Here's how the part is built. I have some questions about the finished solid (model axes, mm). A direction names the side the tool comes from. Give positions to 0.01 mm unless a question says otherwise; leave off trailing zeros. Loops run counter-clockwise (first coordinate to the right, second up) from the corner with the lowest first, then second, coordinate; pieces in that order, holes last. Notation, with made-up numbers: (-21.75, 10.25) -> (8.25, 10.25) arc R15 cw to (8.25, 37.25) -> close; hole circle Ø10 at (11, -9). An arc over 180 degrees is marked (long way). Answer in a Markdown table with one row per item. Add a question column.
Item 1: If I drill on line 1 (X direction, y = -33, z = 5.25); line 2 (X direction, y = -3.5, z = 1); line 3 (Y direction, x = -84, z = 6.55), over which ranges is the centre line in solid material (lowest first)?
Item 2: If we section it at B-B (y = -34): Write out the boundary of the cut face in (x, z), then the cut area to 3 significant figures.
Item 3: For P1, Ø3, axis at x = -84, y = -34, coming from the -Z side; P2, Ø4.5, axis at x = -84, y = 34, coming from the +Z side, each with a flat end and sliding along its axis, tell me the tip position at first contact or that it passes through.
Item 4: If we section it at D-D (x = 40): Write out the boundary of the cut face in (y, z).
Item 5: If we section it at A-A (x = 0): Write out the boundary of the cut face in (y, z).
Item 6: Which directions (+Z, -Z, +X, -X, +Y, -Y) give clear straight access to the entire face, cutting with the end or side of a thin tool? Please do faces 1 (the face through (-81.33, -33.16, 6.03)), 2 (the face through (-37, 21.6, 2)), 3 (the face through (53, 0, 4)).
Item 7: If we section it at C-C (z = 6): Give the number of separate pieces and of enclosed holes in the cut face, then the cut area to 3 significant figures.
Item 8: We'd pull the mould along Y, two halves only. Please class faces 4 (the face through (-1, 1, 8)), 5 (the face through (-84, -36, 4)), 6 (the face through (-1, 38, 4)): released by +Y, released by -Y, zero draft, split by the parting line, or undercut.
```python
from build123d import *

# Parameters (mm, degrees)
SKETCH_1_W          = 176
SKETCH_1_H          = 76
EXTRUDE_1_DEPTH     = 8
SKETCH_2_R          = 1.6
CUT_EXTRUDE_1_DEPTH = 9
SKETCH_2_3_R        = 2.6
CUT_EXTRUDE_2_DEPTH = 3
SKETCH_4_R          = 2.8
CUT_EXTRUDE_3_DEPTH = 4
FILLET_1_R          = 2
SKETCH1_R           = 1.6
CUT_EXTRUDE1_DEPTH  = 9
SKETCH2_R           = 3
CUT_EXTRUDE2_DEPTH  = 4
CUT_EXTRUDE3_DEPTH  = 9


with BuildPart() as part:
    # 草图1 → 凸台-拉伸1 (new body)
    with BuildSketch(Plane.XY):
        Rectangle(SKETCH_1_W, SKETCH_1_H)
    extrude(amount=EXTRUDE_1_DEPTH)

    # 草图2 → 切除-拉伸1 (cut, through all)
    with BuildSketch(Plane(origin=(0, 0, 0), x_dir=(-1, 0, 0), z_dir=(0, 0, -1))):
        with Locations((-84, 34)):
            Circle(SKETCH_2_R)
        with Locations((0, 34)):
            Circle(SKETCH_2_R)
        with Locations((84, 34)):
            Circle(SKETCH_2_R)
        with Locations((-84, -34)):
            Circle(SKETCH_2_R)
        with Locations((84, -34)):
            Circle(SKETCH_2_R)
    extrude(amount=-CUT_EXTRUDE_1_DEPTH, mode=Mode.SUBTRACT)

    # 草图2<3> → 切除-拉伸2 (cut)
    with BuildSketch(Plane(origin=(0, 0, 0), x_dir=(-1, 0, 0), z_dir=(0, 0, -1))):
        with Locations((-84, 0)):
            Circle(SKETCH_2_3_R)
        with Locations((84, 0)):
            Circle(SKETCH_2_3_R)
        with Locations((0, -34)):
            Circle(SKETCH_2_3_R)
    extrude(amount=-CUT_EXTRUDE_2_DEPTH, mode=Mode.SUBTRACT)

    # 草图4 → 切除-拉伸3 (cut)
    with BuildSketch(Plane.XY.offset(8)):
        with Locations((-84, 34)):
            Circle(SKETCH_4_R)
        with Locations((0, 34)):
            Circle(SKETCH_4_R)
        with Locations((-84, -34)):
            Circle(SKETCH_4_R)
        with Locations((84, 34)):
            Circle(SKETCH_4_R)
        with Locations((84, -34)):
            Circle(SKETCH_4_R)
    extrude(amount=-CUT_EXTRUDE_3_DEPTH, mode=Mode.SUBTRACT)

    # 圆角1
    fillet_1_edges = [part.edges().sort_by_distance(p)[0] for p in [
        (-88, 38, 4),
        (88, 38, 4),
        (88, -38, 4),
        (-88, -38, 4),
    ]]
    fillet(fillet_1_edges, radius=FILLET_1_R)

    # Sketch1 → Cut-Extrude1 (cut, through all)
    with BuildSketch(Plane.XY.offset(8)):
        with Locations((-40, 21.5)):
            Circle(SKETCH1_R)
        with Locations((40, 21.5)):
            Circle(SKETCH1_R)
        with Locations((40, -21.5)):
            Circle(SKETCH1_R)
        with Locations((-40, -21.5)):
            Circle(SKETCH1_R)
    extrude(amount=-CUT_EXTRUDE1_DEPTH, mode=Mode.SUBTRACT)

    # Sketch2 → Cut-Extrude2 (cut)
    with BuildSketch(Plane(origin=(0, 0, 0), x_dir=(-1, 0, 0), z_dir=(0, 0, -1))):
        with Locations((-40, 21.5)):
            Circle(SKETCH2_R)
        with Locations((40, 21.5)):
            Circle(SKETCH2_R)
        with Locations((40, -21.5)):
            Circle(SKETCH2_R)
        with Locations((-40, -21.5)):
            Circle(SKETCH2_R)
    extrude(amount=-CUT_EXTRUDE2_DEPTH, mode=Mode.SUBTRACT)

    # Sketch3 → Cut-Extrude3 (cut, through all)
    with BuildSketch(Plane.XY.offset(8)):
        with BuildLine():
            Line((-73, -15), (-73, 15))
            ThreePointArc((-73, 15), (-63, 25), (-53, 15))
            Line((-53, 15), (-53, -15))
            ThreePointArc((-53, -15), (-63, -25), (-73, -15))
        make_face()
        with BuildLine():
            Line((73, -15), (73, 15))
            ThreePointArc((73, 15), (63, 25), (53, 15))
            Line((53, 15), (53, -15))
            ThreePointArc((53, -15), (63, -25), (73, -15))
        make_face()
    extrude(amount=-CUT_EXTRUDE3_DEPTH, mode=Mode.SUBTRACT)


solid = part.part
```
Recorded:
| question | item | result |
|---|---|---|
| 1 | line 1 | x = -88 to -86.62, -81.38 to 81.38, 86.62 to 88 |
| 1 | line 2 | x = -88 to -73, -53 to 53, 73 to 88 |
| 1 | line 3 | y = -38 to -36.8, -31.2 to 31.2, 36.8 to 38 |
| 2 | outline | (-88, 0) -> (-85.6, 0) -> (-85.6, 4) -> (-86.8, 4) -> (-86.8, 8) -> (-88, 8) -> close; (-82.4, 0) -> (-2.6, 0) -> (-2.6, 3) -> (2.6, 3) -> (2.6, 0) -> (82.4, 0) -> (82.4, 4) -> (81.2, 4) -> (81.2, 8) -> (-81.2, 8) -> (-81.2, 4) -> (-82.4, 4) -> close; (85.6, 0) -> (88, 0) -> (88, 8) -> (86.8, 8) -> (86.8, 4) -> (85.6, 4) -> close |
| 2 | area | 1,320 mm^2 |
| 3 | P1 | passes through |
| 3 | P2 | stops at z = 4 |
| 4 | outline | (-38, 0) -> (-24.5, 0) -> (-24.5, 4) -> (-23.1, 4) -> (-23.1, 8) -> (-38, 8) -> close; (-19.9, 4) -> (-18.5, 4) -> (-18.5, 0) -> (18.5, 0) -> (18.5, 4) -> (19.9, 4) -> (19.9, 8) -> (-19.9, 8) -> close; (23.1, 4) -> (24.5, 4) -> (24.5, 0) -> (38, 0) -> (38, 8) -> (23.1, 8) -> close |
| 5 | outline | (-38, 0) -> (-36.6, 0) -> (-36.6, 3) -> (-31.4, 3) -> (-31.4, 0) -> (32.4, 0) -> (32.4, 4) -> (31.2, 4) -> (31.2, 8) -> (-38, 8) -> close; (35.6, 0) -> (38, 0) -> (38, 8) -> (36.8, 8) -> (36.8, 4) -> (35.6, 4) -> close |
| 6 | face 1 | +Z |
| 6 | face 2 | -Z |
| 6 | face 3 | +Z, -Z |
| 7 | separate pieces | 1 |
| 7 | enclosed holes | 11 |
| 7 | area | 11,400 mm^2 |
| 8 | face 4 | zero draft |
| 8 | face 5 | undercut |
| 8 | face 6 | released by +Y |
